```python
from build123d import *

# Parameters (mm, degrees)
SKETCH1_R                = 21.95
BOSS_EXTRUDE1_DEPTH      = 2.34
SKETCH2_R                = 10.925
BOSS_EXTRUDE2_DEPTH      = 4.14
BOSS_EXTRUDE2_DEPTH_BACK = 22.94
SKETCH3_R                = 2.75
CUT_EXTRUDE1_DEPTH       = 7.48
CIRPATTERN1_COUNT        = 3
SKETCH4_R                = 9.725
SKETCH4_R_2              = 8.025
SKETCH4_R_3              = 5.025
SKETCH4_R_4              = 4.525
CUT_EXTRUDE2_DEPTH       = 1.65
SKETCH5_R                = 3.9
BOSS_EXTRUDE3_DEPTH      = 8.9
FILLET1_R                = 1


with BuildPart() as part:
    # Sketch1 → Boss-Extrude1 (new body)
    with BuildSketch(Plane(origin=(0, 0, 0), x_dir=(1, 0, 0), z_dir=(0, 1, 0))):
        Circle(SKETCH1_R)
    extrude(amount=BOSS_EXTRUDE1_DEPTH)

    # Sketch2 → Boss-Extrude2 (add, two sides)
    with BuildSketch(Plane(origin=(0, 2.34, 0), x_dir=(1, 0, 0), z_dir=(0, 1, 0))) as boss_extrude2_sk:
        Circle(SKETCH2_R)
    extrude(amount=BOSS_EXTRUDE2_DEPTH)
    extrude(boss_extrude2_sk.sketch, amount=-BOSS_EXTRUDE2_DEPTH_BACK)

    # Sketch3 → Cut-Extrude1 (cut, through all)
    with BuildSketch(Plane.XZ):
        with Locations((0, 17.475)):
            Circle(SKETCH3_R)
    cut_extrude1 = extrude(amount=-CUT_EXTRUDE1_DEPTH, mode=Mode.SUBTRACT)

    # CirPattern1: Cut-Extrude1 ×3 about axis
    cirpattern1_axis = Axis((0, 0, 0), (0, 1, 0))
    for i in range(1, CIRPATTERN1_COUNT):
        add(cut_extrude1.rotate(cirpattern1_axis, i * 360 / CIRPATTERN1_COUNT), mode=Mode.SUBTRACT)

    # Sketch4 → Cut-Extrude2 (cut)
    with BuildSketch(Plane(origin=(0, 6.48, 0), x_dir=(1, 0, 0), z_dir=(0, 1, 0))):
        Circle(SKETCH4_R)
        Circle(SKETCH4_R_2, mode=Mode.SUBTRACT)
        Circle(SKETCH4_R_3)
        Circle(SKETCH4_R_4, mode=Mode.SUBTRACT)
    extrude(amount=-CUT_EXTRUDE2_DEPTH, mode=Mode.SUBTRACT)

    # Sketch5 → Boss-Extrude3 (add)
    with BuildSketch(Plane(origin=(0, 6.48, 0), x_dir=(1, 0, 0), z_dir=(0, 1, 0))):
        Circle(SKETCH5_R)
    extrude(amount=BOSS_EXTRUDE3_DEPTH)

    # Fillet1
    fillet1_edges = [part.edges().sort_by_distance(p)[0] for p in [
        (-3.9, 15.38, 0),
    ]]
    fillet(fillet1_edges, radius=FILLET1_R)


solid = part.part
```
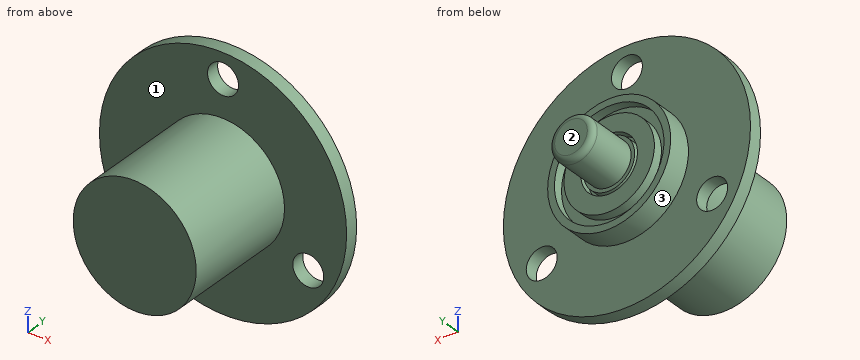
Geometry: final body of the model. Coordinates: model frame, mm. Face numbers are marked on the shaded views. A direction names the side the tool comes from. Coordinates: 2 decimals unless noted, no trailing zeros. Order: outer loops, then holes, each group sorted by start corner. A loop starts at its lowest first (then second) coordinate and runs counter-clockwise, first axis right, second up. Notation, with made-up numbers: (10.25, 43) -> (33.25, 43) arc R23 ccw to (33.25, 63) -> close; hole circle Ø1 at (5.25, -6). An arc over 180 degrees is marked (long way). Write item = value, one per line.
(1) Line query: line 1 (Z direction, x = 0, y = 5.8) (3 decimals); line 2 (Y direction, x = 7.5, z = 2). Output: solid intervals per line, ascending.
Solved:
line_1 = -10.925 to -9.725, -8.025 to -5.025, -4.525 to 4.525, 5.025 to 8.025, 9.725 to 10.925
line_2 = -20.6 to 6.48
(2) Cut plane B-B on x = -15. Return loops of the section in (y, z).
Solved:
outline = (0, -16.03) -> (2.34, -16.03) -> (2.34, -11.48) -> (0, -11.48) -> close; (0, -5.99) -> (2.34, -5.99) -> (2.34, 16.03) -> (0, 16.03) -> close
(3) Cut plane C-C on y = -16. Return loops of the section in (x, z) (3 decimals).
Solved:
outline = circle Ø21.85 at (0, 0)
(4) Pin query (flat end, axial travel): pin 1 Ø10 at (x, z) = (17.5, -4.5) entering from +Y; pin 2 Ø12 at (x, z) = (-7.5, 9.5) entering from +Y; pin 3 Ø9 at (x, z) = (15.13, -8.74) entering from -Y; pin 4 Ø4.5 at (x, z) = (-15.13, -8.74) entering from +Y. Return the tip coordinate at first contact, or that it passes through.
Solved:
pin_1 = 2.34
pin_2 = 6.48
pin_3 = 0
pin_4 = through
(5) Cut plane A-A on x = 13. Return loops of the section in (y, z), plus the area to 3 significant figures.
Solved:
outline = (0, -17.69) -> (2.34, -17.69) -> (2.34, -10.47) -> (0, -10.47) -> close; (0, -7) -> (2.34, -7) -> (2.34, 17.69) -> (0, 17.69) -> close
area = 74.7 mm²
(6) Cut plane D-D on x = 19. Return loops of the section in (y, z).
Solved:
outline = (0, -10.99) -> (2.34, -10.99) -> (2.34, 10.99) -> (0, 10.99) -> close
(7) Access query for the marked faces 1, 2 and 3. Directions: +Z, -Z, +X, -X, +Y, -Y. A direction counts if a zero-diameter tool reaches every point of the face in a straight line with its end or side. Return the directions, or none.
Solved:
face_1 = -Y
face_2 = +Z, -Z, +X, -X, +Y
face_3 = +Y
